Input: dimensioned drawing with shaded views. Units: mm. Origin: part minimum x, y, z. A direction names the side the tool comes from. Round coordinates to 2 decimals unless told otherwise and drop trailing zeros. Loops run counter-clockwise (first coordinate to the right, second up) from the corner with the lowest first, then second, coordinate; pieces in that order, holes last. Notation, with made-up numbers: (-35, 26) - (-7, 26) arc R8 cw to (-7, 39) - close; hole circle Ø9 at (38.25, 62). An arc over 180 degrees is marked (long way). One line per question, with ' | ' between items. Start each with the question number.
1. Pin query (flat end, axial travel): pin 1 (3 mm diameter, centred on x = 22, z = 60.5, fed in from +Y); pin 2 (2.5 mm diameter, centred on x = 19.3, y = 31.69, fed in from +Z); pin 3 (5 mm diameter, centred on x = 22.5, y = 15.5, fed in from +Z). Return the tip coordinate at first contact, or that it passes through.
2. Cut plane A-A (x = 22). Return loops of the section in (y, z) (1 decimal), then the cut area to 3 significant figures.
3. Cut plane B-B (z = 20.5). Return loops of the section in (x, y) (1 decimal).
4. Cut plane C-C (y = 4.5). Return loops of the section in (x, z) (1 decimal).
5. Access query for the marked faces 1 and 2. Directions: +Z, -Z, +X, -X, +Y, -Y. A direction counts if a zero-diameter tool reaches every point of the face in a straight line with its end or side. Return the directions, or none.
6. Ray query, line 1 (Z direction, x = 6, y = 31.5) (1 decimal); line 2 (Z direction, x = 23.5, y = 23) (1 decimal); line 3 (X direction, y = 9, z = 12). Return the intervals inside material, ascending.
7. Cut plane D-D (z = 65.5). Return loops of the section in (x, y) (1 decimal).
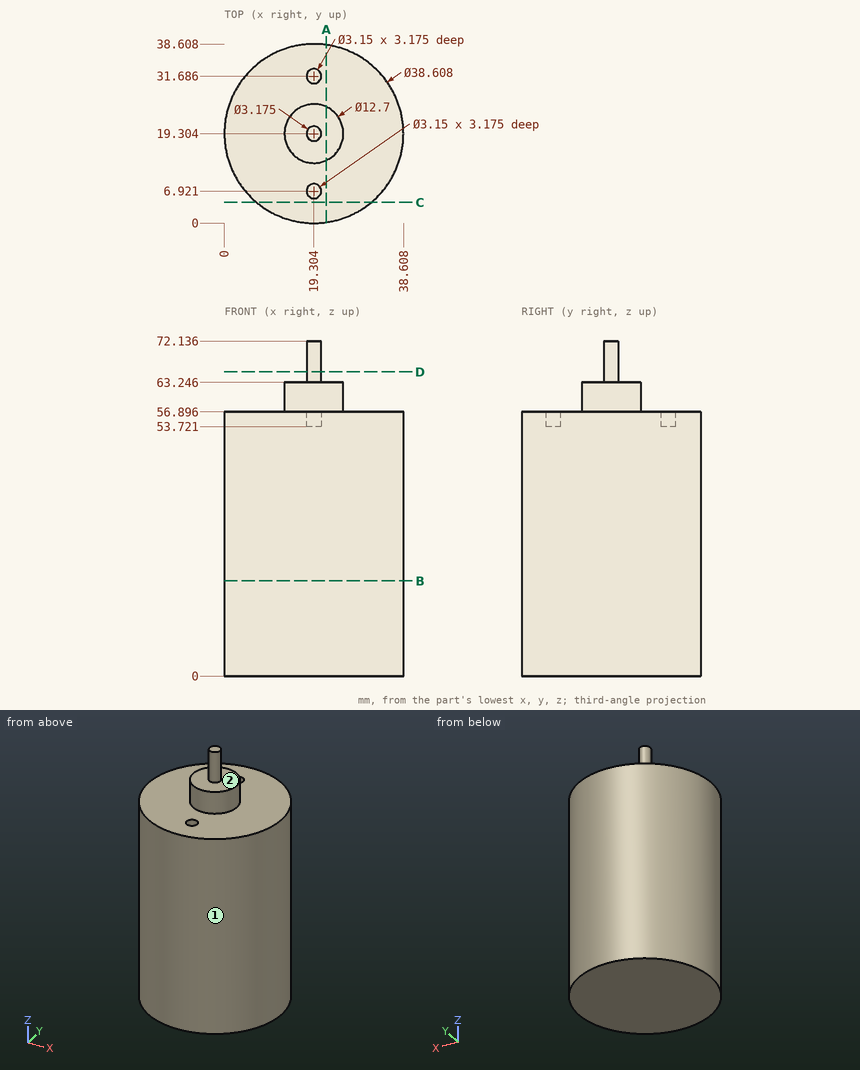
Answers follow:
1) pin 1: stops at y = 25.54 | pin 2: stops at z = 53.72 | pin 3: stops at z = 63.25
2) outline: (0.2, 0) - (38.4, 0) - (38.4, 56.9) - (25.1, 56.9) - (25.1, 63.2) - (13.6, 63.2) - (13.6, 56.9) - (0.2, 56.9) - close | area: 2,250 mm2
3) outline: circle Ø38.6 at (19.3, 19.3)
4) outline: (6.9, 0) - (31.7, 0) - (31.7, 56.9) - (6.9, 56.9) - close
5) face 1: +Z, -Z | face 2: +Z
6) line 1: z = 0 to 56.9 | line 2: z = 0 to 63.2 | line 3: x = 2.98 to 35.63
7) outline: circle Ø3.2 at (19.3, 19.3)
